from build123d import *

# Parameters (mm, degrees)
SKETCH1_W           = 200
SKETCH1_H           = 58
BOSS_EXTRUDE1_DEPTH = 6.25
SKETCH2_R           = 3.5
CUT_EXTRUDE1_DEPTH  = 203.188185857
FILLET1_R           = 24
SKETCH3_R           = 4
CUT_EXTRUDE2_DEPTH  = 10


with BuildPart() as part:
    # Sketch1 → Boss-Extrude1 (new body)
    with BuildSketch(Plane(origin=(0, 0, 0), x_dir=(1, 0, 0), z_dir=(0, 1, 0))):
        with Locations((100, 0)):
            Rectangle(SKETCH1_W, SKETCH1_H)
    extrude(amount=BOSS_EXTRUDE1_DEPTH)

    # Sketch2 → Cut-Extrude1 (cut, through all)
    with BuildSketch(Plane(origin=(0, 0, 0), x_dir=(1, 0, 0), z_dir=(0, 1, 0))):
        with Locations(Location((16, 10, 0), (0, 0, 270))):
            Circle(SKETCH2_R)
        with Locations(Location((16, -10, 0), (0, 0, 270))):
            Circle(SKETCH2_R)
        with BuildLine():
            Line((176, 16), (184, 16))
            ThreePointArc((184, 16), (188, 12), (184, 8))
            Line((184, 8), (176, 8))
            ThreePointArc((176, 8), (172, 12), (176, 16))
        make_face()
        with BuildLine():
            Line((146, 16), (154, 16))
            ThreePointArc((154, 16), (158, 12), (154, 8))
            Line((154, 8), (146, 8))
            ThreePointArc((146, 8), (142, 12), (146, 16))
        make_face()
        with BuildLine():
            Line((146, -8), (154, -8))
            ThreePointArc((154, -8), (158, -12), (154, -16))
            Line((154, -16), (146, -16))
            ThreePointArc((146, -16), (142, -12), (146, -8))
        make_face()
        with BuildLine():
            Line((176, -8), (184, -8))
            ThreePointArc((184, -8), (188, -12), (184, -16))
            Line((184, -16), (176, -16))
            ThreePointArc((176, -16), (172, -12), (176, -8))
        make_face()
    extrude(amount=CUT_EXTRUDE1_DEPTH, mode=Mode.SUBTRACT)

    # Fillet1
    fillet1_edges = [part.edges().sort_by_distance(p)[0] for p in [
        (0, 3.125, -29),
        (0, 3.125, 29),
    ]]
    fillet(fillet1_edges, radius=FILLET1_R)

    # Sketch3 → Cut-Extrude2 (cut)
    with BuildSketch(Plane(origin=(0, 0, 0), x_dir=(1, 0, 0), z_dir=(0, 1, 0))):
        with Locations(Location((66, -10, 0), (0, 0, 270))):
            Circle(SKETCH3_R)
        with Locations(Location((66, 10, 0), (0, 0, 270))):
            Circle(SKETCH3_R)
    extrude(amount=CUT_EXTRUDE2_DEPTH, mode=Mode.SUBTRACT)


solid = part.part
Could you check a few things on this model? Use its own coordinates, in mm. A direction names the side the tool comes from. Give positions to 0.01 mm unless a question says otherwise; leave off trailing zeros. Loops run counter-clockwise (first coordinate to the right, second up) from the corner with the lowest first, then second, coordinate; pieces in that order, holes last. Notation, with made-up numbers: (-12.5, 26.25) -> (42.5, 26.25) arc R24 ccw to (42.5, 50.25) -> close; hole circle Ø3 at (-38.75, -12.5). An arc over 180 degrees is marked (long way). Answer as CSV lines item,"result". Start each with the question number.
(1) Which directions (+Z, -Z, +X, -X, +Y, -Y) give clear straight access to the entire face, cutting with the end or side of a thin tool? Please do faces 1 (the flat face through (99, 6.25, 0)), 2 (the flat face through (150, 3, 8)).
(2) We'd pull the mould along Z, two halves only. Please class faces 3 (the cylindrical face through (6.84, 3.17, 21.78)), 4 (the flat face through (200, 3, 0)), 5 (the flat face through (180, 3, 8)): released by +Z, released by -Z, zero draft, split by the parting line, or undercut.
(3) If we section it at A-A on x = 66: Write out the boundary of the cut face in (y, z).
(4) If we section it at B-B on y = 5.25: Count the separate pieces of the cut face and the enclosed holes in it, then the cut area to 3 significant figures.
(5) I need wall thicknesses on probe 1 along Z at (x, y) = (66, 2.75); probe 2 along Z at (x, y) = (180.5, 0.75); probe 3 along X at (y, z) = (2.5, 10). Which ranges of each line are inside material? Lowest first, please.
(6) If we section it at C-C on z = -10: Write out the boundary of the cut face in (x, y).
(7) If we section it at D-D on x = 16: Write out the boundary of the cut face in (y, z), then the cut area to 3 significant figures.
Computed:
1,face 1,"+Z, -Z, +X, -X, +Y"
1,face 2,"+Y, -Y"
2,face 3,"released by +Z"
2,face 4,"zero draft"
2,face 5,"undercut"
3,outline,"(0, -29) -> (6.25, -29) -> (6.25, -14) -> (0, -14) -> close; (0, -6) -> (6.25, -6) -> (6.25, 6) -> (0, 6) -> close; (0, 14) -> (6.25, 14) -> (6.25, 29) -> (0, 29) -> close"
4,separate pieces,"1"
4,enclosed holes,"8"
4,area,"10,700 mm2"
5,probe 1,"z = -29 to -14, -6 to 6, 14 to 29"
5,probe 2,"z = -29 to -16, -8 to 8, 16 to 29"
5,probe 3,"x = 0.53 to 12.5, 19.5 to 62, 70 to 142.54, 157.46 to 172.54, 187.46 to 200"
6,outline,"(0.53, 0) -> (12.5, 0) -> (12.5, 6.25) -> (0.53, 6.25) -> close; (19.5, 0) -> (62, 0) -> (62, 6.25) -> (19.5, 6.25) -> close; (70, 0) -> (142.54, 0) -> (142.54, 6.25) -> (70, 6.25) -> close; (157.46, 0) -> (172.54, 0) -> (172.54, 6.25) -> (157.46, 6.25) -> close; (187.46, 0) -> (200, 0) -> (200, 6.25) -> (187.46, 6.25) -> close"
7,outline,"(0, -27.63) -> (6.25, -27.63) -> (6.25, -13.5) -> (0, -13.5) -> close; (0, -6.5) -> (6.25, -6.5) -> (6.25, 6.5) -> (0, 6.5) -> close; (0, 13.5) -> (6.25, 13.5) -> (6.25, 27.63) -> (0, 27.63) -> close"
7,area,"258 mm2"
